Verification items for this drawing (mm, ordinates from the low corner). A direction names the side the tool comes from. Coordinates: 2 decimals unless noted, no trailing zeros. Order: outer loops, then holes, each group sorted by start corner. A loop starts at its lowest first (then second) coordinate and runs counter-clockwise, first axis right, second up. Notation, with made-up numbers: M -23,-14.75 L -6,-14.75 A32 cw -6,12.25 Z; hole C 6.25,-34 d11. An arc over 180 degrees is marked long. One line per item, written item: value. Start each with the question number.
1) Sectioned sample at C-C, the plane z = 23.25. Enter the section's corners in (x, y) (3 decimals).
2) Sectioned sample at D-D, the plane x = 6. Enter the section's corners in (y, z), then the cut area to 3 significant figures.
3) Sectioned sample at A-A, the plane z = 8. Enter the section's corners in (x, y).
4) Thickness scan on L1, parallel to Y at x = 10, z = 22.25 (3 decimals); L2, parallel to Y at x = 60, z = 7; L3, parallel to X at y = 22, z = 22.5. Record the ranges inside material, lowest first. Write a range as from..to.
5) Go/stop test with a flat-tipped pin: P1, Ø5, axis at x = 10, y = 37, coming from the +Z side. Record where the tip stops, or that it passes through.
6) Sectioned sample at B-B, the plane y = 6. Enter the section's corners in (x, z) (3 decimals), then the cut area to 3 significant figures.
7) Draft check along X on the marked faces 3, 4 and 5. Enter one of: pulls with the +X half, pulls with the -X half, needs draft (parallel to the pull), parting line crosses it, or undercut.
8) Access from +Z, -Z, +X, -X, +Y, -Y to the whole of each face (thin tool, end or side, straight path). Record for the marked faces 1 and 2.
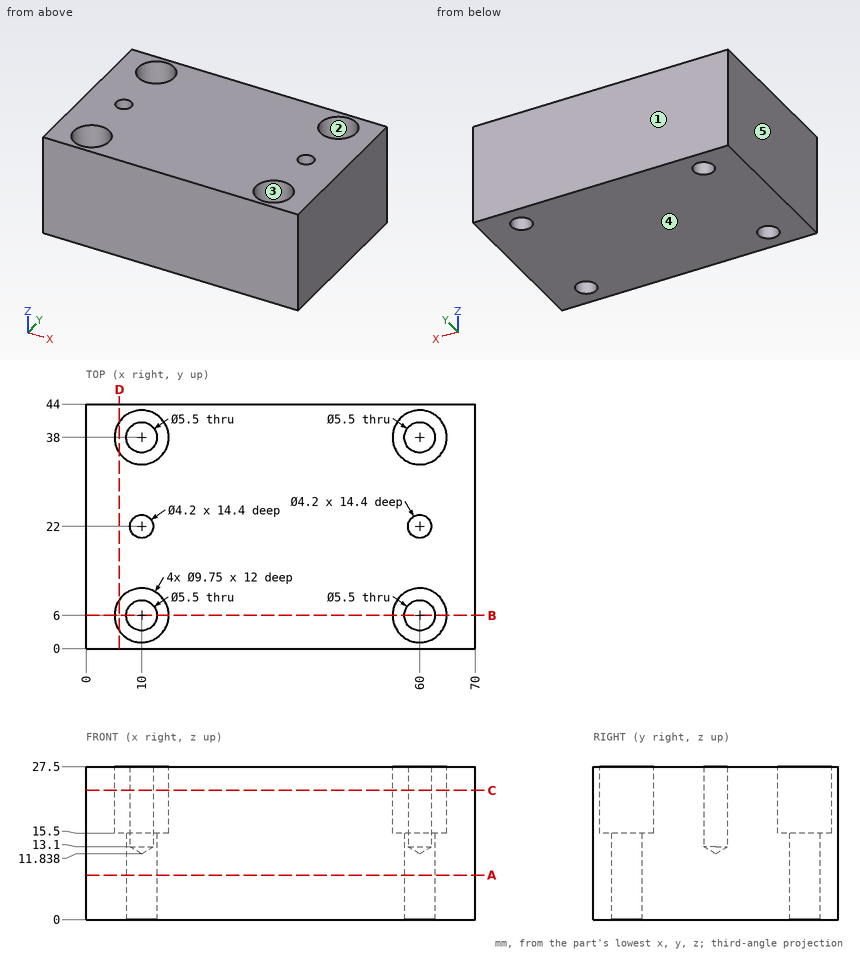
Final values:
1. outline: M 0,0 L 70,0 L 70,44 L 0,44 Z; hole C 10,6 d9.75; hole C 10,38 d9.75; hole C 10,22 d4.2; hole C 60,6 d9.75; hole C 60,38 d9.75; hole C 60,22 d4.2
2. outline: M 0,0 L 44,0 L 44,27.5 L 40.79,27.5 L 40.79,15.5 L 35.21,15.5 L 35.21,27.5 L 8.79,27.5 L 8.79,15.5 L 3.21,15.5 L 3.21,27.5 L 0,27.5 Z
2. area: 1,080 mm^2
3. outline: M 0,0 L 70,0 L 70,44 L 0,44 Z; hole C 10,6 d5.5; hole C 10,38 d5.5; hole C 60,6 d5.5; hole C 60,38 d5.5
4. L1: y = 0..1.125, 10.875..19.9, 24.1..33.125, 42.875..44
4. L2: y = 0..3.25, 8.75..35.25, 40.75..44
4. L3: x = 0..7.9, 12.1..57.9, 62.1..70
5. P1: stops at z = 15.5
6. outline: M 0,0 L 7.25,0 L 7.25,15.5 L 5.125,15.5 L 5.125,27.5 L 0,27.5 Z; M 12.75,0 L 57.25,0 L 57.25,15.5 L 55.125,15.5 L 55.125,27.5 L 14.875,27.5 L 14.875,15.5 L 12.75,15.5 Z; M 62.75,0 L 70,0 L 70,27.5 L 64.875,27.5 L 64.875,15.5 L 62.75,15.5 Z
6. area: 1,520 mm^2
7. face 3: undercut
7. face 4: needs draft
7. face 5: pulls with the -X half
8. face 1: +Z, -Z, +X, -X, +Y
8. face 2: +Z
